Design review of the part built by this model. Coordinates are the model's own, in mm. Face numbers are marked on the shaded views. A direction names the side the tool comes from. Coordinates: 2 decimals unless noted, no trailing zeros. Loops run counter-clockwise (first coordinate to the right, second up) from the corner with the lowest first, then second, coordinate; pieces in that order, holes last. Notation, with made-up numbers: M 18.5,17 L 67.5,17 A20 ccw 67.5,45 Z; hole C 84.5,42 d5. An arc over 180 degrees is marked long. One line per item, written item: value.
Autodesk Inventor part; units mm, degrees
ref_plane "YZ Plane" through (0, 0, 0) normal (1, 0, 0) x (0, 1, 0)
ref_plane "XZ Plane" through (0, 0, 0) normal (0, 1, 0) x (-1, 0, 0)
ref_plane "XY Plane" through (0, 0, 0) normal (0, 0, 1) x (1, 0, 0)
sketch "Sketch1" plane through (0, 0, 0) normal (0, 0, 1) x (1, 0, 0)
  line L0 (-19, 19) -> (19, 19)
  line L1 (19, 19) -> (19, -19)
  line L2 (19, -19) -> (-19, -19)
  line L3 (-19, -19) -> (-19, 19)
  line L4 (-19, 19) -> (19, -19) construction
  line L5 (19, 19) -> (-19, -19) construction
  circle A0 centre (0, 0) radius 4.5
  dimension "d0" = 38
  dimension "d1" = 38
  dimension "d2" = 9
extrude "Extrusion1" add sketch "Sketch1" along normal mid plane 11.64
sketch "Sketch4" plane through (0, 0, 5.82) normal (0, 0, 1) x (1, 0, 0)
  line L0 (-11.25, -11.25) -> (11.25, -11.25) construction
  line L1 (11.25, -11.25) -> (11.25, 11.25) construction
  line L2 (11.25, 11.25) -> (-11.25, 11.25) construction
  line L3 (-11.25, 11.25) -> (-11.25, -11.25) construction
  line L4 (-11.25, -11.25) -> (11.25, 11.25) construction
  line L5 (11.25, -11.25) -> (-11.25, 11.25) construction
  point P0 (0, 0)
  point P1 (-7, -7)
  point P2 (0, 0)
  point P3 (0, 0)
  point P4 (-7, 7)
  point P5 (7, -7)
  point P6 (7, 7)
  dimension "d17" = 22.5
  dimension "d18" = 22.5
  dimension "d47" = 7
  dimension "d48" = 7
  dimension "d51" = 14
  dimension "d54" = 14
sketch "Sketch5" plane through (0, 0, -5.82) normal (0, 0, -1) x (-1, 0, 0)
  circle A0 centre (0, 0) radius 4.5
  circle A1 centre (0, 0) radius 15.24
  dimension "d19" = 30.48
extrude "Extrusion2" cut sketch "Sketch5" against normal blind 8.64 contours A0 | A1
sketch "Sketch6" plane through (-19, 19, 5.82) normal (0, 1, 0) x (1, 0, 0)
  line L0 (0, 11.64) -> (38, 11.64)
  line L1 (3.76, 3) -> (34.24, 3)
  line L2 (10, 11.64) -> (28, 11.64)
  line L3 (28, 11.64) -> (28, 3)
  line L4 (28, 3) -> (10, 3)
  line L5 (10, 3) -> (10, 11.64)
  line L6 (0, 11.64) -> (0, 0)
  line L7 (38, 11.64) -> (38, 0)
  point P0 (19, 5.82)
  point P1 (10, 3)
  dimension "d22" = 10
  dimension "d23" = 10
extrude "Extrusion3" cut sketch "Sketch6" against normal through all
sketch "Sketch7" plane through (19, -19, 5.82) normal (1, 0, 0) x (0, 0, -1)
  line L0 (11.64, 31.2987) -> (11.64, 6.7013)
  line L1 (3, 31.2987) -> (3, 6.7013)
  line L2 (11.64, 28) -> (3, 28)
  line L3 (3, 28) -> (3, 10)
  line L4 (3, 10) -> (11.64, 10)
  line L5 (11.64, 10) -> (11.64, 28)
  line L6 (11.64, 38) -> (0, 38)
  line L7 (11.64, 0) -> (0, 0)
  point P0 (5.82, 19)
  point P1 (11.64, 10)
  point P2 (3, 28)
  dimension "d26" = 10
  dimension "d27" = 10
extrude "Extrusion4" cut sketch "Sketch7" against normal through all
sketch "Sketch8" plane through (0, 0, -5.82) normal (0, 0, -1) x (-1, 0, 0)
  line L0 (-12.2987, -9) -> (-19, -9)
  line L1 (-19, -9) -> (-19, -19)
  line L2 (-19, -19) -> (-9, -19)
  line L3 (-9, -19) -> (-9, -12.2987)
  arc A0 (-12.2987, -9) -> (-9, -12.2987) centre (0, 0) ccw
  point P0 (-15, -15)
  point P1 (-15, 15)
  point P2 (15, -15)
  point P3 (15, 15)
  dimension "d30" = 15
  dimension "d31" = 15
  dimension "d34" = 30
  dimension "d37" = 30
hole "Hole1" at (15, -15, -5.82) at (15, 15, -5.82) at (-15, 15, -5.82) at (-15, -15, -5.82) direction (0, 0, 1) diameter 2.5 depth 4
hole "Hole2" at (-7, -7, 5.82) at (-7, 7, 5.82) at (7, -7, 5.82) at (7, 7, 5.82) direction (0, 0, -1) diameter 1.567 end through all
sketch "Sketch9" plane through (0, 0, 5.82) normal (0, 0, 1) x (1, 0, 0)
  circle A0 centre (15, -15) radius 1.25
  circle A1 centre (-15, -15) radius 1.25
  circle A2 centre (-15, 15) radius 1.25
  circle A3 centre (15, 15) radius 1.25
  point P0 (0, 0)
hole "Hole3" at (15, -15, 5.82) at (-15, -15, 5.82) at (-15, 15, 5.82) at (15, 15, 5.82) direction (0, 0, -1) diameter 2.5 depth 3
equation "\"d1\" = d0"
equation "\"d18\" = d17"
properties part number "pmtbase"
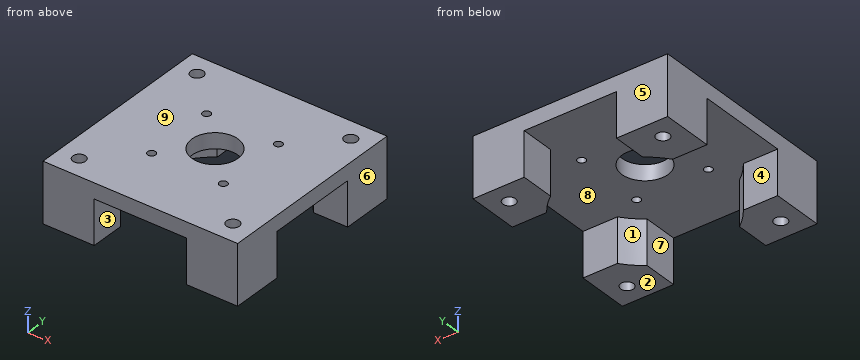
(1) We need section B-B on z = 5. State how many separate pieces and enclosed holes the cut face has, then the cut area to 3 significant figures.
Reply:
separate pieces: 1
enclosed holes: 9
area: 1,350 mm2
(2) To check wall thickness, follow line 1 along Y through (x, z) = (-15, 4.95); line 2 along X through (y, z) = (15, -3.15); line 3 along X through (y, z) = (7, 4.45). State the ranges of each line that lie inside material, in increasing order. Write a range as [from, to].
Reply:
line 1: y = [-19, -16.25], [-13.75, 13.75], [16.25, 19]
line 2: x = [-19, -16.25], [-13.75, -9], [9, 13.75], [16.25, 19]
line 3: x = [-19, -7.78], [-6.22, 6.22], [7.78, 19]
(3) Insertion check: pin 1 (1.5 mm diameter, centred on x = -15, y = 15, fed in from +Z); pin 2 (1.2 mm diameter, centred on x = -14.5, y = -15, fed in from -Z). Each pin has a flat end and moves straight along its axis. Give the tip position at first contact, or say it passes through.
Reply:
pin 1: stops at z = 2.82
pin 2: stops at z = -1.82
(4) We need section A-A on x = 0. State the section outline as (y, z) points.
Reply:
outline: M -19,2.82 L -4.5,2.82 L -4.5,5.82 L -19,5.82 Z; M 4.5,2.82 L 19,2.82 L 19,5.82 L 4.5,5.82 Z
(5) We need section C-C on y = 7. State the section outline as (x, z) points, then the cut area to 3 significant figures.
Reply:
outline: M -19,2.82 L -7.78,2.82 L -7.78,5.82 L -19,5.82 Z; M -6.22,2.82 L 6.22,2.82 L 6.22,5.82 L -6.22,5.82 Z; M 7.78,2.82 L 19,2.82 L 19,5.82 L 7.78,5.82 Z
area: 105 mm2
(6) Mouldability with a two-part tool opening along X and no side actions: class the marked faces 6, 7, 8 and 9 as released by +X, released by -X, zero draft, split by the parting line, or undercut.
Reply:
face 6: released by +X
face 7: undercut
face 8: undercut
face 9: zero draft
(7) Tool access review of the marked faces 1, 2, 3, 4 and 5: name each direction out of +Z, -Z, +X, -X, +Y, -Y from which nothing blocks a thin tool from reaching the whole face with its end or side.
Reply:
face 1: -Z
face 2: -Z, +X, -X, +Y, -Y
face 3: -Z, +Y, -Y
face 4: -Z, +X, -X
face 5: +Z, -Z, +X, -X, +Y
